```python
from build123d import *

# Parameters (mm, degrees)
SKETCH1_W           = 6
SKETCH1_H           = 9
BOSS_EXTRUDE1_DEPTH = 4
SKETCH2_W           = 0.7
SKETCH2_H           = 0.7
BOSS_EXTRUDE2_DEPTH = 5
SKETCH3_W           = 3.5
SKETCH3_H           = 0.314102564
CUT_EXTRUDE1_DEPTH  = 1


with BuildPart() as part:
    # Sketch1 → Boss-Extrude1 (new body)
    with BuildSketch(Plane(origin=(0, 0, 0), x_dir=(1, 0, 0), z_dir=(0, 1, 0))):
        Rectangle(SKETCH1_W, SKETCH1_H)
    extrude(amount=BOSS_EXTRUDE1_DEPTH)

    # Sketch2 → Boss-Extrude2 (add)
    with BuildSketch(Plane.XZ):
        with Locations((-2, 3.5)):
            Rectangle(SKETCH2_W, SKETCH2_H)
        with Locations((0, 3.5)):
            Rectangle(SKETCH2_W, SKETCH2_H)
        with Locations((2, 3.5)):
            Rectangle(SKETCH2_W, SKETCH2_H)
    extrude(amount=BOSS_EXTRUDE2_DEPTH)

    # Sketch3 → Cut-Extrude1 (cut)
    # profile 1 of 2: a face of its own
    with BuildSketch(Plane(origin=(0, 4, 0), x_dir=(1, 0, 0), z_dir=(0, 1, 0))):
        with Locations((0.016516605, 1.480769231)):
            Rectangle(SKETCH3_W, SKETCH3_H)
    # profile 2 of 2: a face of its own
    with BuildSketch(Plane(origin=(0, 4, 0), x_dir=(1, 0, 0), z_dir=(0, 1, 0))):
        with BuildLine():
            Line((1.766516605, 0.560897436), (1.766516605, -0.139523237))
            add(Edge.make_bspline(
                [(1.766516605, -0.139523237), (1.766361019, -0.186264366), (1.766062277, -0.27601251), (1.764396514, -0.40458578), (1.759622158, -0.521412877), (1.755513575, -0.626432717), (1.748021633, -0.719643372), (1.740860986, -0.801330663), (1.731487326, -0.87111836), (1.722781903, -0.913364211), (1.718840323, -0.932491987)],
                knots=[0, 0, 0, 0, 1.410062039, 2.707475311, 3.878576406, 4.937260626, 5.877586885, 6.699081471, 7.410979367, 8, 8, 8, 8], degree=3))
            add(Edge.make_bspline(
                [(1.718840323, -0.932491987), (1.712514276, -0.958099062), (1.699997132, -1.008766944), (1.673527119, -1.081710467), (1.64294591, -1.151248932), (1.606748352, -1.217121383), (1.565565808, -1.27933393), (1.519157663, -1.337793424), (1.467287579, -1.392165635), (1.4112801, -1.442868932), (1.350646542, -1.488829838), (1.286270173, -1.528602989), (1.218553628, -1.562660539), (1.147261096, -1.589849705), (1.072995235, -1.611722556), (0.995107565, -1.627150208), (0.913946279, -1.636401005), (0.858588413, -1.637342914), (0.830519009, -1.637820513)],
                knots=[0, 0, 0, 0, 1.02737288, 2.032829108, 3.019628684, 3.985738875, 4.958353778, 5.924249254, 6.890702889, 7.883913451, 8.865824512, 9.85161466, 10.829249435, 11.81541824, 12.821369441, 13.843154991, 14.906364023, 16, 16, 16, 16], degree=3))
            add(Edge.make_bspline(
                [(0.830519009, -1.637820513), (0.783883851, -1.636351553), (0.692886578, -1.633485231), (0.560826446, -1.606759595), (0.437634391, -1.562985023), (0.323481852, -1.502654559), (0.220533831, -1.425861636), (0.130417059, -1.333574003), (0.05430934, -1.22626297), (0.002092736, -1.125894415), (-0.031505665, -1.037192031), (-0.055264297, -0.963952361), (-0.073311274, -0.883999597), (-0.089713454, -0.798480783), (-0.102229635, -0.706735362), (-0.111118503, -0.608948089), (-0.116834112, -0.50487439), (-0.117669187, -0.433534628), (-0.118098779, -0.396834936)],
                knots=[0, 0, 0, 0, 1.260402266, 2.459371274, 3.627181936, 4.786749125, 5.93865593, 7.087644312, 8.261344208, 9.485713728, 10.136162886, 10.825977872, 11.566646758, 12.35154167, 13.181268117, 14.0701832, 15.007234106, 16, 16, 16, 16], degree=3))
            Line((-0.118098779, -0.396834936), (-1.733483395, -1.682692308))
            Line((-1.733483395, -1.682692308), (-1.733483395, -1.294270833))
            Line((-1.733483395, -1.294270833), (-0.118098779, -0.008413462))
            Line((-0.118098779, -0.008413462), (-0.118098779, 0.246794872))
            Line((-0.118098779, 0.246794872), (-1.733483395, 0.246794872))
            Line((-1.733483395, 0.246794872), (-1.733483395, 0.560897436))
            Line((-1.733483395, 0.560897436), (1.766516605, 0.560897436))
        make_face()
        with BuildLine():
            Line((1.407542246, 0.246794872), (0.24087558, 0.246794872))
            Line((0.24087558, 0.246794872), (0.235967727, -0.394030449))
            add(Edge.make_bspline(
                [(0.235967727, -0.394030449), (0.23595449, -0.423950488), (0.235928834, -0.481944044), (0.239922609, -0.565844711), (0.244465932, -0.643964817), (0.251415263, -0.716005588), (0.260371383, -0.781999101), (0.271574209, -0.841912719), (0.284626785, -0.895843103), (0.304826248, -0.958744454), (0.336846887, -1.02896197), (0.383355041, -1.105368013), (0.442230666, -1.170213186), (0.508484032, -1.226122294), (0.582826418, -1.269186547), (0.661958048, -1.300529767), (0.745195752, -1.320199384), (0.802367596, -1.322537824), (0.831220131, -1.323717949)],
                knots=[0, 0, 0, 0, 1.14660753, 2.222451964, 3.218720504, 4.145691244, 4.995719623, 5.770487122, 6.480909919, 7.121111896, 8.299844659, 9.430703709, 10.534634535, 11.641396424, 12.741395289, 13.810956493, 14.895269934, 16, 16, 16, 16], degree=3))
            add(Edge.make_bspline(
                [(0.831220131, -1.323717949), (0.85937451, -1.322534196), (0.915166216, -1.320188431), (0.996619653, -1.300491656), (1.074046514, -1.268684245), (1.145970993, -1.224082893), (1.211802985, -1.170189), (1.267351902, -1.106181988), (1.313870883, -1.035285329), (1.343381026, -0.968975107), (1.361509576, -0.909746951), (1.37425074, -0.858314844), (1.384573588, -0.799980074), (1.392599408, -0.734882443), (1.399821729, -0.663139722), (1.40450449, -0.584555466), (1.407334752, -0.499220423), (1.407471472, -0.440073241), (1.407542246, -0.409455128)],
                knots=[0, 0, 0, 0, 1.100801541, 2.181386982, 3.260112282, 4.364594493, 5.481957178, 6.577424609, 7.668452592, 8.790448866, 9.403819393, 10.091598921, 10.863153553, 11.720938239, 12.658472417, 13.685008818, 14.801622349, 16, 16, 16, 16], degree=3))
            Line((1.407542246, -0.409455128), (1.407542246, 0.246794872))
        make_face(mode=Mode.SUBTRACT)
    extrude(amount=-CUT_EXTRUDE1_DEPTH, mode=Mode.SUBTRACT)


solid = part.part
```
The model under review builds one solid part; all positions refer to its coordinate system, in mm. A direction names the side the tool comes from. Give positions to 0.01 mm unless a question says otherwise; leave off trailing zeros. Write each loop counter-clockwise with the first axis right and the second up, starting at its lowest first coordinate (ties: lowest second). Pieces come first, ordered by that corner, then holes. Notation, with made-up numbers: (6, 35) -> (10, 35) arc R6 cw to (10, 43) -> close; hole circle Ø2 at (86, 25). An arc over 180 degrees is marked (long way). Answer in a Markdown table with one row per item.
1) Mouldability with a two-part tool opening along Z and no side actions: class faces 3 (the flat face through (0, 2, -4.5)), 4 (the flat face through (1, 4, 1)), 5 (the flat face through (-0.937, 3.507, 0.66)) as +Z half, -Z half, draft (parallel to the pull), parting line (faces both ways), or undercut.
Worked answers:
| item | result |
|---|---|
| face 3 | -Z half |
| face 4 | draft |
| face 5 | undercut |
2) Add section C-C on z = -3. State the section outline as (x, y) points, plus the area to 3 significant figures.
Worked answers:
| item | result |
|---|---|
| outline | (-3, 0) -> (3, 0) -> (3, 4) -> (-3, 4) -> close |
| area | 24.0 mm² |
3) Tool access review of faces 1 (the flat face through (0.8, 3.5, -0.247)), 2 (the flat face through (0, 2, 4.5)): name each direction out of +Z, -Z, +X, -X, +Y, -Y from which nothing blocks a thin tool from reaching the whole face with its end or side.
Worked answers:
| item | result |
|---|---|
| face 1 | +Y |
| face 2 | +Z, +X, -X, +Y, -Y |
4) Clearance check with flat-ended pins moving along their axes: P1, Ø0.8, axis at x = 2, y = -2.5, coming from the +Z side; P2, Ø0.6, axis at y = -2.5, z = 3.5, coming from the +X side; P3, Ø3, axis at x = 1, z = -3.5, coming from the -Y side. State where each tip first meets the part, or that it passes through.
Worked answers:
| item | result |
|---|---|
| P1 | z = 3.85 |
| P2 | x = 2.35 |
| P3 | y = 0 |
5) Add section B-B on x = -2. State the section outline as (y, z) points.
Worked answers:
| item | result |
|---|---|
| outline | (-5, 3.15) -> (0, 3.15) -> (0, -4.5) -> (4, -4.5) -> (4, 4.5) -> (0, 4.5) -> (0, 3.85) -> (-5, 3.85) -> close |
6) Add section A-A on y = -0.25. State the section outline as (x, z) points.
Worked answers:
| item | result |
|---|---|
| outline | (-2.35, 3.15) -> (-1.65, 3.15) -> (-1.65, 3.85) -> (-2.35, 3.85) -> close; (-0.35, 3.15) -> (0.35, 3.15) -> (0.35, 3.85) -> (-0.35, 3.85) -> close; (1.65, 3.15) -> (2.35, 3.15) -> (2.35, 3.85) -> (1.65, 3.85) -> close |
7) For L1, parallel to X at y = -2.5, z = 3.75; L2, parallel to Z at x = 0.5, y = 3.25; L3, parallel to Y at x = 0.5, z = -0.5, list the stretches that pass through material, from the lowest coordinate up. Write a range as [from, to].
Worked answers:
| item | result |
|---|---|
| L1 | [-2.35, -1.65], [-0.35, 0.35], [1.65, 2.35] |
| L2 | [-4.5, -1.64], [-1.32, -0.56], [-0.25, 1.22], [1.58, 4.5] |
| L3 | [0, 3] |
8) Add section D-D on x = -0.5. State the section outline as (y, z) points.
Worked answers:
| item | result |
|---|---|
| outline | (0, -4.5) -> (4, -4.5) -> (4, -1.64) -> (3, -1.64) -> (3, -1.32) -> (4, -1.32) -> (4, -0.56) -> (3, -0.56) -> (3, -0.25) -> (4, -0.25) -> (4, 0.31) -> (3, 0.31) -> (3, 0.7) -> (4, 0.7) -> (4, 4.5) -> (0, 4.5) -> close |
